from build123d import *

# Parameters (mm, degrees)
SKETCH1_W           = 25
SKETCH1_H           = 12
SKETCH1_R           = 4.05
BOSS_EXTRUDE1_DEPTH = 3
SKETCH2_W           = 4
SKETCH2_H           = 12
BOSS_EXTRUDE2_DEPTH = 5


with BuildPart() as part:
    # Sketch1 → Boss-Extrude1 (new body)
    with BuildSketch(Plane(origin=(0, 0, 0), x_dir=(1, 0, 0), z_dir=(0, 1, 0))):
        Rectangle(SKETCH1_W, SKETCH1_H)
        with Locations(Location((0, 0, 0), (0, 0, 270))):
            Circle(SKETCH1_R, mode=Mode.SUBTRACT)
    extrude(amount=BOSS_EXTRUDE1_DEPTH)

    # Sketch2 → Boss-Extrude2 (add)
    with BuildSketch(Plane(origin=(0, 3, 0), x_dir=(1, 0, 0), z_dir=(0, 1, 0))):
        with Locations((-10.5, 0)):
            Rectangle(SKETCH2_W, SKETCH2_H)
        with Locations((10.5, 0)):
            Rectangle(SKETCH2_W, SKETCH2_H)
    extrude(amount=BOSS_EXTRUDE2_DEPTH)


solid = part.part
Model file for the job. Use its own axes, mm. A direction names the side the tool comes from. Coordinates: 2 decimals unless noted, no trailing zeros. Write each loop counter-clockwise with the first axis right and the second up, starting at its lowest first coordinate (ties: lowest second). Pieces come first, ordered by that corner, then holes. Notation, with made-up numbers: (19, 5.5) -> (56, 5.5) arc R11 cw to (56, 19.5) -> close; hole circle Ø8 at (-16, 72.5). An arc over 180 degrees is marked (long way). One line per item, written item: value. Start each with the question number.
1) Slice it at D-D on z = 5.25. Write the cut outline in (x, y), then the cut area to 3 significant figures.
2) Slice it at A-A on z = 0. Write the cut outline in (x, y), then the cut area to 3 significant figures.
3) Probe probe 1 along X at (y, z) = (1.55, 0); probe 2 along X at (y, z) = (5.5, -4.5); probe 3 along Y at (x, z) = (-7.75, 0.25). List the from-to ranges inside material, lowest first.
4) Pull direction Z, two halves, no side cores. Call faces 3 (the face through (8.5, 5, 0)), 4 (the face through (-3.593, 1.479, 1.869)), 5 (the face through (0, 2, -6)): +Z half, -Z half, draft (parallel to the pull), parting line (faces both ways), or undercut.
5) Slice it at C-C on y = 3.5. Write the cut outline in (x, z), then the cut area to 3 significant figures.
6) Flat gauge pin, fed straight in: pin 1 Ø4 at (x, z) = (-1.5, 3.5) entering from +Y. Where does the tip first touch, or does it go through?
7) Which spindle directions (+Z, -Z, +X, -X, +Y, -Y) get a long thin tool onto all of the face, cutting with end or side? Do faces 1 (the face through (-2, 3, -4)), 2 (the face through (-3, 0, -4)). Say none if no direction does.
8) Slice it at B-B on x = 0. Write the cut outline in (y, z).
Answers follow:
1. outline: (-12.5, 0) -> (12.5, 0) -> (12.5, 8) -> (8.5, 8) -> (8.5, 3) -> (-8.5, 3) -> (-8.5, 8) -> (-12.5, 8) -> close
1. area: 115 mm2
2. outline: (-12.5, 0) -> (-4.05, 0) -> (-4.05, 3) -> (-8.5, 3) -> (-8.5, 8) -> (-12.5, 8) -> close; (4.05, 0) -> (12.5, 0) -> (12.5, 8) -> (8.5, 8) -> (8.5, 3) -> (4.05, 3) -> close
2. area: 90.7 mm2
3. probe 1: -12.5 to -4.05, 4.05 to 12.5
3. probe 2: -12.5 to -8.5, 8.5 to 12.5
3. probe 3: 0 to 3
4. face 3: draft
4. face 4: undercut
4. face 5: -Z half
5. outline: (-12.5, -6) -> (-8.5, -6) -> (-8.5, 6) -> (-12.5, 6) -> close; (8.5, -6) -> (12.5, -6) -> (12.5, 6) -> (8.5, 6) -> close
5. area: 96.0 mm2
6. pin 1: y = 3
7. face 1: +Z, -Z, +Y
7. face 2: +Z, -Z, +X, -X, -Y
8. outline: (0, -6) -> (3, -6) -> (3, -4.05) -> (0, -4.05) -> close; (0, 4.05) -> (3, 4.05) -> (3, 6) -> (0, 6) -> close
